Check sheet for the modelled part. Datum: model origin and axes. Units: mm. Face numbers are marked on the shaded views. A direction names the side the tool comes from. Give positions to 0.01 mm unless a question says otherwise; leave off trailing zeros. Write each loop counter-clockwise with the first axis right and the second up, starting at its lowest first coordinate (ties: lowest second). Pieces come first, ordered by that corner, then holes. Notation, with made-up numbers: M 85.5,13 L 114.5,13 A17 cw 114.5,45 Z; hole C 9.25,46.5 d6. An arc over 180 degrees is marked long. One line per item, written item: value. Start each with the question number.
from build123d import *

# Parameters (mm, degrees)
F0_R     = 1.25
F1_DEPTH = 2
F3_DEPTH = 1
F5_R     = 1


# Not quite as in the source:
# - a pattern or mirror of a feature is missing from the dataset's text; its kind, count and spacing are read off the source's solid


with BuildPart() as f1:
    # F0 (on Right) → F1 (new body)
    with BuildSketch(Plane.YZ):
        with BuildLine():
            ThreePointArc((-2, 0), (0, -2), (2, 0))
            ThreePointArc((2, 0), (0, 2), (-2, 0))
        make_face()
        Circle(F0_R, mode=Mode.SUBTRACT)
        with BuildLine():
            Line((2, -5), (2, 0))
            ThreePointArc((2, 0), (0, -2), (-2, 0))
            Line((-2, 0), (-2, -5))
            ThreePointArc((-2, -5), (0, -3), (2, -5))
        make_face()
        with BuildLine():
            ThreePointArc((-2, -5), (0, -7), (2, -5))
            Line((2, -5), (-2, -5))
        make_face()
        with BuildLine():
            Line((-2, -5), (2, -5))
            ThreePointArc((2, -5), (0, -3), (-2, -5))
        make_face()
    extrude(amount=-F1_DEPTH)

    # F2 (on face) → F3 (join)
    with BuildSketch(Plane(origin=(-2, 0, 0), x_dir=(0, -1, 0), z_dir=(-1, 0, 0))):
        with BuildLine():
            ThreePointArc((0, -2), (-1, -1.7320508076), (-1.7320508076, -1))
            Line((-1.7320508076, -1), (-2, -1))
            Line((-2, -1), (-2, -4))
            Line((-2, -4), (-1.7320508076, -4))
            ThreePointArc((-1.7320508076, -4), (-1, -3.2679491924), (0, -3))
            Line((0, -3), (2, -3))
            Line((2, -3), (2, -2))
            Line((2, -2), (0, -2))
        make_face()
        with BuildLine():
            Line((-1.7320508076, -4), (-2, -4))
            Line((-2, -4), (-2, -5))
            ThreePointArc((-2, -5), (0, -7), (2, -5))
            Line((2, -5), (2, -3))
            Line((2, -3), (0, -3))
            ThreePointArc((0, -3), (-1, -3.2679491924), (-1.7320508076, -4))
        make_face()
    f3 = extrude(amount=F3_DEPTH)

    # F3_copies: F3 across plane
    add(f3.mirror(Plane(origin=(-1, 0, 0), x_dir=(0, 0, 1), z_dir=(1, 0, 0))))

    # F5
    f5_edges = [f1.edges().sort_by_distance(p)[0] for p in [
        (-3, 2, -3),
        (-3, -2, -3.5),
        (-3, 0, -7),
        (1, 0, -7),
        (1, 2, -3),
        (1, -2, -3.5),
    ]]
    fillet(f5_edges, radius=F5_R)


solid = f1.part
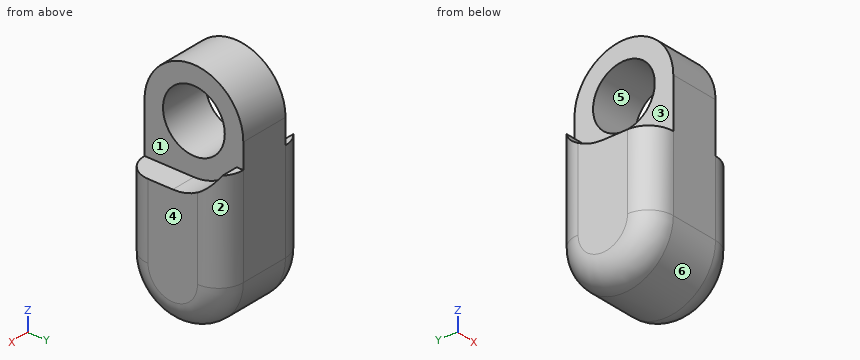
1) Material ranges on L1, parallel to Z at x = -0.9, y = 0; L2, parallel to X at y = -0.4, z = -1.25; L3, parallel to Z at x = -1.6, y = 0.65, recorded low to high. Write a range as from..to.
2) Tool access check on the marked faces 1, 2 and 3. Record the directions out of +Z, -Z, +X, -X, +Y, -Y that give a thin tool (end or side, any length) a straight path to the whole face; none if there is none.
3) Cross-section at A-A (z = 0.25). Record the boundary of the cut face in (x, y).
4) Cross-section at B-B (x = -0.6). Record the boundary of the cut face in (y, z).
5) Gauge pin test, flat ends, axial feed: pin 1 (2 mm diameter, centred on y = 0.5, z = 0.5, fed in from -X); pin 2 (1 mm diameter, centred on x = -0.5, y = -1, fed in from +Z); pin 3 (0.5 mm diameter, centred on x = 0.5, y = -1, fed in from +Z). Record the tip position at first contact, or that the pin passes through.
6) Draft check along Z on the marked faces 4, 5 and 6. Enter one of: released by +Z, released by -Z, zero draft, split by the parting line, or undercut.
7) Cross-section at C-C (z = -2.75). Record the boundary of the cut face in (x, y).
Data:
1. L1: z = -7..-1.25, 1.25..2
1. L2: x = -2..0
1. L3: z = -6.89..-1.07, 1.07..1.89
2. face 1: +Z, +X, -Y
2. face 2: +Z, -Z, +X, +Y
2. face 3: +Z, -X, -Y
3. outline: M -2,-1.98 L 0,-1.98 L 0,-1.22 L -2,-1.22 Z; M -2,1.22 L 0,1.22 L 0,1.98 L -2,1.98 Z
4. outline: M -2,-5 A2 ccw 2,-5 L 2,0 A2 ccw -2,0 Z; hole C 0,0 d2.5
5. pin 1: stops at x = -2
5. pin 2: stops at z = 1.94
5. pin 3: stops at z = -2
6. face 4: zero draft
6. face 5: undercut
6. face 6: released by -Z
7. outline: M -3,-1 A1 ccw -2,-2 L 0,-2 A1 ccw 1,-1 L 1,1 A1 ccw 0,2 L -2,2 A1 ccw -3,1 Z
